Geometry check sheet. Reference: the model listing, model coordinates, mm. Face numbers are marked on the shaded views. A direction names the side the tool comes from. Coordinates: 2 decimals unless noted, no trailing zeros. Order: outer loops, then holes, each group sorted by start corner. A loop starts at its lowest first (then second) coordinate and runs counter-clockwise, first axis right, second up. Notation, with made-up numbers: M 6.5,-35.5 L 25.5,-35.5 A18 ccw 25.5,-0.5 Z; hole C 37.25,36.5 d4. An arc over 180 degrees is marked long. One line per item, written item: value. Start each with the question number.
1) Go/stop test with flat-tipped pins: P1, Ø4, axis at y = 19.5, z = 44.5, coming from the +X side; P2, Ø15, axis at y = 14, z = 74, coming from the -X side; P3, Ø4, axis at x = 70, z = 75.5, coming from the +Y side; P4, Ø5.5, axis at x = 6.35, z = 68.58, coming from the -Y side. Record where each tip stops, or that it passes through.
2) Access from +Z, -Z, +X, -X, +Y, -Y to the whole of each face (thin tool, end or side, straight path). Record for the marked faces 1 and 2.
3) Sectioned sample at D-D, the plane x = 6.35. State how many separate pieces and enclosed holes the cut face has, then the cut area to 3 significant figures.
4) Sectioned sample at C-C, the plane x = 69.85. Enter the section's corners in (y, z), then the cut area to 3 significant figures.
5) Thickness scan on L1, parallel to X at y = 16, z = 104.5; L2, parallel to X at y = 2.05, z = 88.9; L3, parallel to Z at x = 38.5, y = 23. Record the ranges inside material, lowest first. Write a range as from..to.
6) Sectioned sample at B-B, the plane z = 107.95. Enter the section's corners in (x, y), then the cut area to 3 significant figures.
7) Sectioned sample at A-A, the plane z = 25.4. Enter the section's corners in (x, y) (3 decimals).
8) Draft check along X on the marked faces 3, 4 and 5. Enter one of: pulls with the +X half, pulls with the -X half, needs draft (parallel to the pull), parting line crosses it, or undercut.
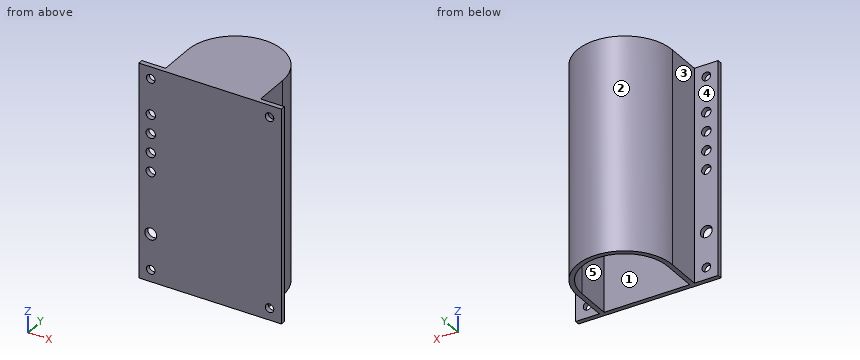
```python
from build123d import *

# Parameters (mm, degrees)
BOSS_EXTRUDE2_DEPTH = 114.3
SKETCH2_R           = 2.286
CUT_EXTRUDE1_DEPTH  = 145.383975911
CUT_EXTRUDE2_DEPTH  = 114.046
SKETCH5_R           = 2.499999953
CUT_EXTRUDE3_DEPTH  = 146.186053394
SKETCH7_R           = 3.175
CUT_EXTRUDE4_DEPTH  = 145.383975911


with BuildPart() as part:
    # Sketch1 → Boss-Extrude2 (new body)
    with BuildSketch(Plane.XY):
        with BuildLine():
            Line((0, 0), (76.2, 0))
            Line((76.2, 0), (76.2, 2.54))
            Line((76.2, 2.54), (63.5, 2.54))
            Line((63.5, 2.54), (63.5, 21.59))
            ThreePointArc((63.5, 21.59), (38.1, 46.99), (12.7, 21.59))
            Line((12.7, 21.59), (12.7, 2.54))
            Line((12.7, 2.54), (0, 2.54))
            Line((0, 2.54), (0, 0))
        make_face()
    extrude(amount=BOSS_EXTRUDE2_DEPTH)

    # Sketch2 → Cut-Extrude1 (cut, through all)
    with BuildSketch(Plane(origin=(0, 2.54, 0), x_dir=(1, 0, 0), z_dir=(0, 1, 0))):
        with Locations(Location((6.35, -6.35, 0), (0, 0, 270))):
            Circle(SKETCH2_R)
        with Locations(Location((69.85, -6.35, 0), (0, 0, 270))):
            Circle(SKETCH2_R)
        with Locations(Location((69.85, -107.95, 0), (0, 0, 270))):
            Circle(SKETCH2_R)
        with Locations(Location((6.35, -107.95, 0), (0, 0, 270))):
            Circle(SKETCH2_R)
    extrude(amount=-CUT_EXTRUDE1_DEPTH, mode=Mode.SUBTRACT)

    # Sketch4 → Cut-Extrude2 (cut)
    with BuildSketch(Plane(origin=(0, 0, 0), x_dir=(-1, 0, 0), z_dir=(0, 0, -1))):
        with BuildLine():
            Line((-60.96, 2.54), (-15.24, 2.54))
            Line((-15.24, 2.54), (-15.24, 21.59))
            ThreePointArc((-15.24, 21.59), (-38.1, 44.45), (-60.96, 21.59))
            Line((-60.96, 21.59), (-60.96, 2.54))
        make_face()
    extrude(amount=-CUT_EXTRUDE2_DEPTH, mode=Mode.SUBTRACT)

    # Sketch5 → Cut-Extrude3 (cut, through all)
    with BuildSketch(Plane(origin=(0, 0, 0), x_dir=(-1, 0, 0), z_dir=(0, -1, 0))):
        with Locations(Location((-6.35, -88.9, 0), (0, 0, 90))):
            Circle(SKETCH5_R)
        with Locations(Location((-6.35, -78.74, 0), (0, 0, 90))):
            Circle(SKETCH5_R)
        with Locations(Location((-6.35, -68.58, 0), (0, 0, 90))):
            Circle(SKETCH5_R)
        with Locations(Location((-6.35, -58.42, 0), (0, 0, 90))):
            Circle(SKETCH5_R)
    extrude(amount=-CUT_EXTRUDE3_DEPTH, mode=Mode.SUBTRACT)

    # Sketch7 → Cut-Extrude4 (cut, through all)
    with BuildSketch(Plane(origin=(0, 2.54, 0), x_dir=(1, 0, 0), z_dir=(0, 1, 0))):
        with Locations(Location((6.35, -25.4, 0), (0, 0, 270))):
            Circle(SKETCH7_R)
    extrude(amount=-CUT_EXTRUDE4_DEPTH, mode=Mode.SUBTRACT)


solid = part.part
```
Final values:
1. P1: stops at x = 63.5
1. P2: stops at x = 12.7
1. P3: stops at y = 2.54
1. P4: stops at y = 0
2. face 1: -Z
2. face 2: +Z, -Z, +Y
3. separate pieces: 8
3. enclosed holes: 0
3. area: 200 mm^2
4. outline: M 0,0 L 2.54,0 L 2.54,4.06 L 0,4.06 Z; M 0,8.64 L 2.54,8.64 L 2.54,105.66 L 0,105.66 Z; M 0,110.24 L 2.54,110.24 L 2.54,114.3 L 0,114.3 Z
4. area: 267 mm^2
5. L1: x = 12.7..15.24, 60.96..63.5
5. L2: x = 0..3.85, 8.85..76.2
5. L3: z = 114.05..114.3
6. outline: M 0,0 L 4.06,0 L 4.06,2.54 L 0,2.54 Z; M 8.64,0 L 67.56,0 L 67.56,2.54 L 63.5,2.54 L 63.5,21.59 A25.4 ccw 12.7,21.59 L 12.7,2.54 L 8.64,2.54 Z; M 72.14,0 L 76.2,0 L 76.2,2.54 L 72.14,2.54 Z; hole M 15.24,2.54 L 60.96,2.54 L 60.96,21.59 A22.86 ccw 15.24,21.59 Z
6. area: 460 mm^2
7. outline: M 0,0 L 3.175,0 L 3.175,2.54 L 0,2.54 Z; M 9.525,0 L 76.2,0 L 76.2,2.54 L 63.5,2.54 L 63.5,21.59 A25.4 ccw 12.7,21.59 L 12.7,2.54 L 9.525,2.54 Z; hole M 15.24,2.54 L 60.96,2.54 L 60.96,21.59 A22.86 ccw 15.24,21.59 Z
8. face 3: pulls with the -X half
8. face 4: needs draft
8. face 5: undercut
